Geometry check sheet. Reference: the model listing, model coordinates, mm. Round coordinates to 2 decimals unless told otherwise and drop trailing zeros. Use a Markdown table: item, result.
```python
from build123d import *

# Parameters (mm, degrees)
SKETCH1_R           = 2.1463
BOSS_EXTRUDE1_DEPTH = 187.5
SKETCH2_W           = 61.526977309
SKETCH2_H           = 152.756633319
CUT_EXTRUDE1_DEPTH  = 20.9898


with BuildPart() as part:
    # Sketch1 → Boss-Extrude1 (new body, symmetric)
    with BuildSketch(Plane.XY):
        with BuildLine():
            Line((-9.9949, 7.9883), (-9.9949, 3.2893))
            ThreePointArc((-9.9949, 3.2893), (-9.76427588, 2.73252412), (-9.2075, 2.5019))
            Line((-9.2075, 2.5019), (-8.4963, 2.5019))
            ThreePointArc((-8.4963, 2.5019), (-8.280773853, 2.591173853), (-8.1915, 2.8067))
            Line((-8.1915, 2.8067), (-8.1915, 4.9149))
            ThreePointArc((-8.1915, 4.9149), (-7.674065253, 5.689295824), (-6.760603096, 5.507596904))
            Line((-6.760603096, 5.507596904), (-4.505765747, 3.252759555))
            ThreePointArc((-4.505765747, 3.252759555), (-3.856054457, 2.280397894), (-3.627906192, 1.133419111))
            Line((-3.627906192, 1.133419111), (-3.627906192, -1.133419111))
            ThreePointArc((-3.627906192, -1.133419111), (-3.856054457, -2.280397894), (-4.505765747, -3.252759555))
            Line((-4.505765747, -3.252759555), (-6.760603096, -5.507596904))
            ThreePointArc((-6.760603096, -5.507596904), (-7.674065253, -5.689295824), (-8.1915, -4.9149))
            Line((-8.1915, -4.9149), (-8.1915, -2.8067))
            ThreePointArc((-8.1915, -2.8067), (-8.280773853, -2.591173853), (-8.4963, -2.5019))
            Line((-8.4963, -2.5019), (-9.2075, -2.5019))
            ThreePointArc((-9.2075, -2.5019), (-9.76427588, -2.73252412), (-9.9949, -3.2893))
            Line((-9.9949, -3.2893), (-9.9949, -7.9883))
            ThreePointArc((-9.9949, -7.9883), (-9.407180467, -9.407180467), (-7.9883, -9.9949))
            Line((-7.9883, -9.9949), (-3.2893, -9.9949))
            ThreePointArc((-3.2893, -9.9949), (-2.73252412, -9.76427588), (-2.5019, -9.2075))
            Line((-2.5019, -9.2075), (-2.5019, -8.4963))
            ThreePointArc((-2.5019, -8.4963), (-2.591173853, -8.280773853), (-2.8067, -8.1915))
            Line((-2.8067, -8.1915), (-4.9149, -8.1915))
            ThreePointArc((-4.9149, -8.1915), (-5.689295824, -7.674065253), (-5.507596904, -6.760603096))
            Line((-5.507596904, -6.760603096), (-3.252759555, -4.505765747))
            ThreePointArc((-3.252759555, -4.505765747), (-2.280397894, -3.856054457), (-1.133419111, -3.627906192))
            Line((-1.133419111, -3.627906192), (1.133419111, -3.627906192))
            ThreePointArc((1.133419111, -3.627906192), (2.280397894, -3.856054457), (3.252759555, -4.505765747))
            Line((3.252759555, -4.505765747), (5.507596904, -6.760603096))
            ThreePointArc((5.507596904, -6.760603096), (5.689295824, -7.674065253), (4.9149, -8.1915))
            Line((4.9149, -8.1915), (2.8067, -8.1915))
            ThreePointArc((2.8067, -8.1915), (2.591173853, -8.280773853), (2.5019, -8.4963))
            Line((2.5019, -8.4963), (2.5019, -9.2075))
            ThreePointArc((2.5019, -9.2075), (2.73252412, -9.76427588), (3.2893, -9.9949))
            Line((3.2893, -9.9949), (7.9883, -9.9949))
            ThreePointArc((7.9883, -9.9949), (9.407180467, -9.407180467), (9.9949, -7.9883))
            Line((9.9949, -7.9883), (9.9949, -3.2893))
            ThreePointArc((9.9949, -3.2893), (9.76427588, -2.73252412), (9.2075, -2.5019))
            Line((9.2075, -2.5019), (8.4963, -2.5019))
            ThreePointArc((8.4963, -2.5019), (8.280773853, -2.591173853), (8.1915, -2.8067))
            Line((8.1915, -2.8067), (8.1915, -4.9149))
            ThreePointArc((8.1915, -4.9149), (7.674065253, -5.689295824), (6.760603096, -5.507596904))
            Line((6.760603096, -5.507596904), (4.505765747, -3.252759555))
            ThreePointArc((4.505765747, -3.252759555), (3.856054457, -2.280397894), (3.627906192, -1.133419111))
            Line((3.627906192, -1.133419111), (3.627906192, 1.133419111))
            ThreePointArc((3.627906192, 1.133419111), (3.856054457, 2.280397894), (4.505765747, 3.252759555))
            Line((4.505765747, 3.252759555), (6.760603096, 5.507596904))
            ThreePointArc((6.760603096, 5.507596904), (7.674065253, 5.689295824), (8.1915, 4.9149))
            Line((8.1915, 4.9149), (8.1915, 2.8067))
            ThreePointArc((8.1915, 2.8067), (8.280773853, 2.591173853), (8.4963, 2.5019))
            Line((8.4963, 2.5019), (9.2075, 2.5019))
            ThreePointArc((9.2075, 2.5019), (9.76427588, 2.73252412), (9.9949, 3.2893))
            Line((9.9949, 3.2893), (9.9949, 7.9883))
            ThreePointArc((9.9949, 7.9883), (9.407180467, 9.407180467), (7.9883, 9.9949))
            Line((7.9883, 9.9949), (3.2893, 9.9949))
            ThreePointArc((3.2893, 9.9949), (2.73252412, 9.76427588), (2.5019, 9.2075))
            Line((2.5019, 9.2075), (2.5019, 8.4963))
            ThreePointArc((2.5019, 8.4963), (2.591173853, 8.280773853), (2.8067, 8.1915))
            Line((2.8067, 8.1915), (4.9149, 8.1915))
            ThreePointArc((4.9149, 8.1915), (5.689295824, 7.674065253), (5.507596904, 6.760603096))
            Line((5.507596904, 6.760603096), (3.252759555, 4.505765747))
            ThreePointArc((3.252759555, 4.505765747), (2.280397894, 3.856054457), (1.133419111, 3.627906192))
            Line((1.133419111, 3.627906192), (-1.133419111, 3.627906192))
            ThreePointArc((-1.133419111, 3.627906192), (-2.280397894, 3.856054457), (-3.252759555, 4.505765747))
            Line((-3.252759555, 4.505765747), (-5.507596904, 6.760603096))
            ThreePointArc((-5.507596904, 6.760603096), (-5.689295824, 7.674065253), (-4.9149, 8.1915))
            Line((-4.9149, 8.1915), (-2.8067, 8.1915))
            ThreePointArc((-2.8067, 8.1915), (-2.591173853, 8.280773853), (-2.5019, 8.4963))
            Line((-2.5019, 8.4963), (-2.5019, 9.2075))
            ThreePointArc((-2.5019, 9.2075), (-2.73252412, 9.76427588), (-3.2893, 9.9949))
            Line((-3.2893, 9.9949), (-7.9883, 9.9949))
            ThreePointArc((-7.9883, 9.9949), (-9.407180467, 9.407180467), (-9.9949, 7.9883))
        make_face()
        Circle(SKETCH1_R, mode=Mode.SUBTRACT)
    extrude(amount=BOSS_EXTRUDE1_DEPTH, both=True)

    # Sketch2 → Cut-Extrude1 (cut, through all)
    with BuildSketch(Plane(origin=(0, 9.9949, 0), x_dir=(1, 0, 0), z_dir=(0, 1, 0))):
        with Locations((5.480851427, 136.37831666)):
            Rectangle(SKETCH2_W, SKETCH2_H)
    extrude(amount=-CUT_EXTRUDE1_DEPTH, mode=Mode.SUBTRACT)


solid = part.part
```
Item 1: Mould release check, pull along Y, two halves, no side actions. Record for faces 1 (the face through (2.05, 0.64, 62.02)), 2 (the face through (-0.1, 2.4, -60)), 3 (the face through (-6, 9.995, 65)), 4 (the face through (6, -9.995, 65)): +Y half, -Y half, draft (parallel to the pull), parting line (faces both ways), or undercut.
Outcome:
| item | result |
|---|---|
| face 1 | undercut |
| face 2 | draft |
| face 3 | +Y half |
| face 4 | -Y half |
Item 2: Go/stop test with flat-tipped pins: pin 1 (0.7 mm diameter, centred on x = -0.5, z = 60, fed in from +Y); pin 2 (0.7 mm diameter, centred on y = 0.5, z = 92, fed in from +X); pin 3 (0.7 mm diameter, centred on y = 0, z = 125, fed in from -X). Record where each tip stops, or that it passes through.
Outcome:
| item | result |
|---|---|
| pin 1 | stops at y = 3.63 |
| pin 2 | stops at x = 3.63 |
| pin 3 | stops at x = -3.63 |
Item 3: Material ranges on line 1 along Y through (x, z) = (4.5, -37); line 2 along Y through (x, z) = (6.75, 100), recorded low to high. Write a range as from..to.
Outcome:
| item | result |
|---|---|
| line 1 | y = -9.99..-8.19, -5.75..-3.25, 3.25..5.75, 8.19..9.99 |
| line 2 | y = -9.99..-5.5, 5.5..9.99 |
